```python
from build123d import *

# Parameters (mm, degrees)
F0_W      = 584.2
F0_H      = 584.2
F1_DEPTH  = 25.4
F2_W      = 25.4
F2_H      = 304.8
F3_DEPTH  = 1016
F4_W      = 304.8
F4_H      = 25.4
F5_DEPTH  = 1016
F6_W      = 27.716884
F6_H      = 304.8
F7_DEPTH  = 1016
F8_W      = 306.838674
F8_H      = 25.4
F9_DEPTH  = 1016
F10_W     = 25.4
F10_H     = 279.4
F11_DEPTH = 711.2
F12_W     = 584.2
F12_H     = 25.4
F13_DEPTH = 711.2
F14_W     = 25.4
F14_H     = 584.2
F15_DEPTH = 711.2
F16_W     = 279.4
F16_H     = 25.4
F17_DEPTH = 711.2


with BuildPart() as f1:
    # F0 (on Top) → F1 (new body)
    with BuildSketch(Plane.XY):
        with Locations((-12.97821, 67.926513)):
            Rectangle(F0_W, F0_H)
    extrude(amount=F1_DEPTH)

    # F2 (on face) → F3 (join)
    with BuildSketch(Plane.XY.offset(25.4)):
        with Locations((266.42179, 207.626513)):
            Rectangle(F2_W, F2_H)
    extrude(amount=F3_DEPTH)

    # F4 (on face) → F5 (join)
    with BuildSketch(Plane.XY.offset(25.4)):
        with Locations((124.683116, 349.342086)):
            Rectangle(F4_W, F4_H)
    extrude(amount=F5_DEPTH)

    # F6 (on face) → F7 (join)
    with BuildSketch(Plane.XY.offset(25.4)):
        with Locations((-13.858442, 207.626513)):
            Rectangle(F6_W, F6_H)
    extrude(amount=F7_DEPTH)

    # F8 (on face) → F9 (join)
    with BuildSketch(Plane.XY.offset(25.4)):
        with Locations((125.702453, 67.926513)):
            Rectangle(F8_W, F8_H)
    extrude(amount=F9_DEPTH)

    # F10 (on face) → F11 (join)
    with BuildSketch(Plane.XY.offset(25.4)):
        with Locations((266.42179, -84.473487)):
            Rectangle(F10_W, F10_H)
    extrude(amount=F11_DEPTH)

    # F12 (on face) → F13 (join)
    with BuildSketch(Plane.XY.offset(25.4)):
        with Locations((-12.97821, -211.473487)):
            Rectangle(F12_W, F12_H)
    extrude(amount=F13_DEPTH)

    # F14 (on face) → F15 (join)
    with BuildSketch(Plane.XY.offset(25.4)):
        with Locations((-292.37821, 67.926513)):
            Rectangle(F14_W, F14_H)
    extrude(amount=F15_DEPTH)

    # F16 (on face) → F17 (join)
    with BuildSketch(Plane.XY.offset(25.4)):
        with Locations((-167.416884, 347.326513)):
            Rectangle(F16_W, F16_H)
    extrude(amount=F17_DEPTH)


solid = f1.part
```
Geometry check sheet. Reference: the model listing, model coordinates, mm. A direction names the side the tool comes from. Round coordinates to 2 decimals unless told otherwise and drop trailing zeros. Loops run counter-clockwise (first coordinate to the right, second up) from the corner with the lowest first, then second, coordinate; pieces in that order, holes last. Notation, with made-up numbers: M 8,17.25 L 15,17.25 A18 ccw 15,40.25 Z; hole C 78,46.25 d8. An arc over 180 degrees is marked long. Return JSON: item names as keys, results as strings. Group by question number.
(1) Set-up check for faces 4 (the face through (123, 362.042, 526)), 5 (the face through (125, 336.642, 526)), 6 (the face through (-81, -212, 736.6)): record each of +Z, -Z, +X, -X, +Y, -Y from which the full face is reachable in a straight line by a thin tool's end or side.
(2) Go/stop test with flat-tipped pins: pin 1 (1 mm diameter, centred on y = -118.5, z = 143.5, fed in from -X); pin 2 (1 mm diameter, centred on x = -306, y = 349.5, fed in from -Z); pin 3 (1.6 mm diameter, centred on y = 361, z = 292.5, fed in from +X). Record where each tip stops, or that it passes through.
(3) Section check D-D, the plane z = 832.5. Enter the section's corners in (x, y), and give its area (3 significant figures).
(4) Scan lines: line 1 along Y through (x, z) = (219, 599); line 2 along Y through (x, z) = (-35.5, 135.5); line 3 along X through (y, z) = (303, 668.5). Record each from-to range of solid material in increasing order. Write a range as [from, to].
(5) Section check A-A, the plane z = 710.5. Enter the section's corners in (x, y), and give its area (3 significant figures).
(6) Section check B-B, the plane x = -168.5. Enter the section's corners in (y, z), and give its area (3 significant figures).
(7) Section check C-C, the plane y = -32. Enter the section's corners in (x, z).
(8) Mould release check, pull along X, two halves, no side actions. Record for faces 1 (the face through (124, 55.227, 526)), 2 (the face through (279.122, 64, 398)), 3 (the face through (-17, 72, 0)): pulls with the +X half, pulls with the -X half, needs draft (parallel to the pull), parting line crosses it, or undercut.
Data:
{
 "1": {"face 4": "+Z, -Z, +X, -X, +Y", "face 5": "+Z", "face 6": "+Z, -X, -Y"},
 "2": {"pin 1": "x = -305.08", "pin 2": "z = 25.4", "pin 3": "x = 277.08"},
 "3": {"outline": "M -27.72,55.23 L 279.12,55.23 L 279.12,360.03 L 277.08,360.03 L 277.08,362.04 L -27.72,362.04 Z; hole M 0,80.63 L 253.72,80.63 L 253.72,336.64 L 0,336.64 Z", "area": "29,200 mm²"},
 "4": {"line 1": "[-224.17, -198.77], [55.23, 80.63], [336.64, 362.04]", "line 2": "[-224.17, -198.77], [334.63, 360.03]", "line 3": "[-305.08, -279.68], [-27.72, 0], [253.72, 279.12]"},
 "5": {"outline": "M -307.12,334.63 L -305.08,334.63 L -305.08,-224.17 L 279.12,-224.17 L 279.12,360.03 L 277.08,360.03 L 277.08,362.04 L -27.72,362.04 L -27.72,360.03 L -307.12,360.03 Z; hole M -279.68,-198.77 L 253.72,-198.77 L 253.72,55.23 L -27.72,55.23 L -27.72,334.63 L -279.68,334.63 Z; hole M 0,80.63 L 253.72,80.63 L 253.72,336.64 L 0,336.64 Z", "area": "71,100 mm²"},
 "6": {"outline": "M -224.17,0 L 360.03,0 L 360.03,736.6 L 334.63,736.6 L 334.63,25.4 L -198.77,25.4 L -198.77,736.6 L -224.17,736.6 Z", "area": "51,000 mm²"},
 "7": {"outline": "M -305.08,0 L 279.12,0 L 279.12,736.6 L 253.72,736.6 L 253.72,25.4 L -279.68,25.4 L -279.68,736.6 L -305.08,736.6 Z"},
 "8": {"face 1": "undercut", "face 2": "pulls with the +X half", "face 3": "needs draft"}
}
